Geometry: see drawing. Coordinates: mm, zero at the bounding-box minimum. Coordinates: 2 decimals unless noted, no trailing zeros. Order: outer loops, then holes, each group sorted by start corner. A loop starts at its lowest first (then second) coordinate and runs counter-clockwise, first axis right, second up. Notation, with made-up numbers: (54.25, -11.75) -> (63.25, -11.75) arc R21 cw to (63.25, 4.25) -> close; hole circle Ø7 at (38.5, -14). An arc over 180 degrees is marked (long way). One line per item, written item: value. Start each with the question number.
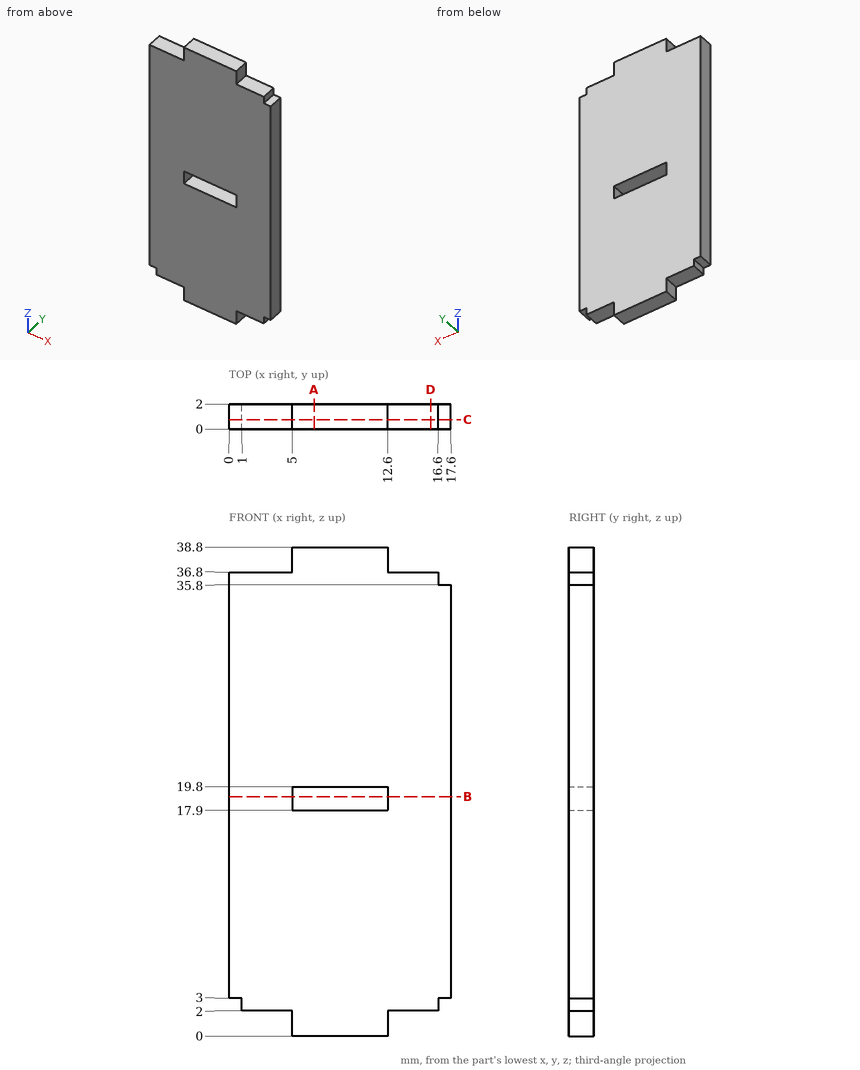
1) Pin query (flat end, axial travel): pin 1 Ø0.6 at (x, y) = (15.5, 1.5) entering from -Z; pin 2 Ø1.1 at (x, y) = (17.5, 1) entering from +Z; pin 3 Ø0.8 at (x, y) = (0.5, 1) entering from -Z. Return the tip coordinate at first contact, or that it passes through.
2) Ray query, line 1 along Z through (x, y) = (11.5, 0.5); line 2 along Z through (x, y) = (16.75, 0.45); line 3 along Z through (x, y) = (15.75, 1.5). Return the intervals inside material, ascending. Write a range as from..to.
3) Section query A-A, the plane x = 6.75. Return the cut outline in (y, z).
4) Section query B-B, the plane z = 19. Return the cut outline in (x, y), plus the area to 3 significant figures.
5) Section query D-D, the plane x = 16. Return the cut outline in (y, z).
6) Section query C-C, the plane y = 0.75. Return the cut outline in (x, z), plus the area to 3 significant figures.
Entries:
1. pin 1: stops at z = 2
1. pin 2: stops at z = 35.8
1. pin 3: stops at z = 3
2. line 1: z = 0..17.9, 19.8..38.8
2. line 2: z = 3..35.8
2. line 3: z = 2..36.8
3. outline: (0, 0) -> (2, 0) -> (2, 17.9) -> (0, 17.9) -> close; (0, 19.8) -> (2, 19.8) -> (2, 38.8) -> (0, 38.8) -> close
4. outline: (0, 0) -> (5, 0) -> (5, 2) -> (0, 2) -> close; (12.6, 0) -> (17.6, 0) -> (17.6, 2) -> (12.6, 2) -> close
4. area: 20.0 mm2
5. outline: (0, 2) -> (2, 2) -> (2, 36.8) -> (0, 36.8) -> close
6. outline: (0, 3) -> (1, 3) -> (1, 2) -> (5, 2) -> (5, 0) -> (12.6, 0) -> (12.6, 2) -> (16.6, 2) -> (16.6, 3) -> (17.6, 3) -> (17.6, 35.8) -> (16.6, 35.8) -> (16.6, 36.8) -> (12.6, 36.8) -> (12.6, 38.8) -> (5, 38.8) -> (5, 36.8) -> (0, 36.8) -> close; hole (5, 17.9) -> (12.6, 17.9) -> (12.6, 19.8) -> (5, 19.8) -> close
6. area: 625 mm2
